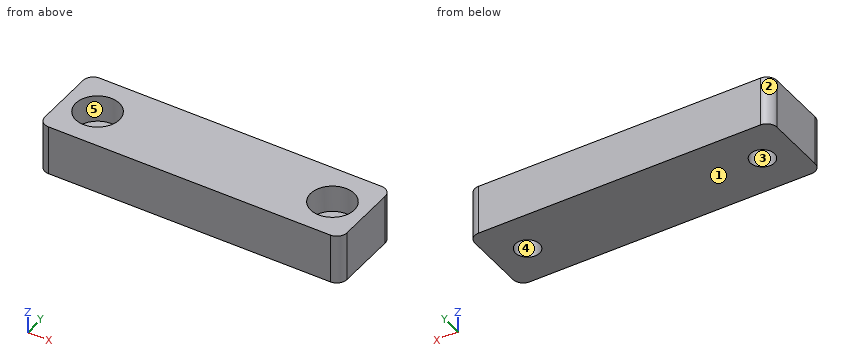
Solid Edge part; units mm, degrees
sketch "Sketch1" plane through (0, 0, 0) normal (0, 0, 1) x (1, 0, 0)
  line L0 (-22.5, 6) -> (-22.5, -6)
  line L1 (-22.5, -6) -> (22.5, -6)
  line L2 (22.5, -6) -> (22.5, 6)
  line L3 (22.5, 6) -> (-22.5, 6)
extrude "Protrusion1" add sketch "Sketch1" along normal blind 7.4
hole "Hole_1" at (17.5, 0, 7.4) direction (0, 0, -1) diameter 3.6 end through all counterbore diameter 6.5 counterbore depth 4
hole "Hole1" at (-17.5, 0, 7.4) direction (0, 0, -1) diameter 3.6 end through all counterbore diameter 6.5 counterbore depth 4
fillet "Round_1" radius 1.5 4 edges at (-22.5, -6, 3.7) (22.5, -6, 3.7) (22.5, 6, 3.7) (-22.5, 6, 3.7)
properties material "Acrylic, high impact grade"
Here's how the part is built. I have some questions about the finished solid (model axes, mm). Face numbers are marked on the shaded views. A direction names the side the tool comes from. Give positions to 0.01 mm unless a question says otherwise; leave off trailing zeros. Loops run counter-clockwise (first coordinate to the right, second up) from the corner with the lowest first, then second, coordinate; pieces in that order, holes last. Notation, with made-up numbers: M 61.5,-24 L 116.5,-24 A17 cw 116.5,-12 Z; hole C 25.5,73.5 d2. An arc over 180 degrees is marked long. Return JSON: item names as keys, results as strings.
Item 1: Imagine slicing it at C-C on x = 17.5. List the corners of the cut face in (y, z) for me, then the cut area to 3 significant figures.
A:
{"outline": "M -6,0 L -1.8,0 L -1.8,3.4 L -3.25,3.4 L -3.25,7.4 L -6,7.4 Z; M 1.8,0 L 6,0 L 6,7.4 L 3.25,7.4 L 3.25,3.4 L 1.8,3.4 Z", "area": "50.6 mm^2"}
Item 2: On a 3-axis mill with a long thin cutter (end or side, diameter ignored), from which of +Z, -Z, +X, -X, +Y, -Y can I reach the whole of each face in a straight line? I mean the marked faces 4 and 5. Say none if no direction works.
A:
{"face 4": "+Z, -Z", "face 5": "+Z"}
Item 3: I'm going to push flat-ended pins straight in: pin 1 Ø3 at (x, y) = (-17.5, 0) entering from +Z; pin 2 Ø4 at (x, y) = (-17.5, 0) entering from +Z. Where does each tip first touch, or does it pass through?
A:
{"pin 1": "passes through", "pin 2": "stops at z = 3.4"}
Item 4: Please list where these lines run through material, in increasing order: line 1 (X direction, y = 0, z = 4.5); line 2 (X direction, y = 0, z = 1.55); line 3 (Y direction, x = -17.5, z = 1.5).
A:
{"line 1": "x = -22.5 to -20.75, -14.25 to 14.25, 20.75 to 22.5", "line 2": "x = -22.5 to -19.3, -15.7 to 15.7, 19.3 to 22.5", "line 3": "y = -6 to -1.8, 1.8 to 6"}
Item 5: Thinking about a two-plate mould opening in Y: for the marked faces 1, 2 and 3, which applies, released by +Y, released by -Y, zero draft, split by the parting line, or undercut?
A:
{"face 1": "zero draft", "face 2": "released by +Y", "face 3": "undercut"}
Item 6: Imagine slicing it at D-D on z = 5. List the corners of the cut face in (x, y) for me.
A:
{"outline": "M -22.5,-4.5 A1.5 ccw -21,-6 L 21,-6 A1.5 ccw 22.5,-4.5 L 22.5,4.5 A1.5 ccw 21,6 L -21,6 A1.5 ccw -22.5,4.5 Z; hole C -17.5,0 d6.5; hole C 17.5,0 d6.5"}
Item 7: Imagine slicing it at B-B on z = 2.5. List the corners of the cut face in (x, y) for me, then the cut area to 3 significant figures.
A:
{"outline": "M -22.5,-4.5 A1.5 ccw -21,-6 L 21,-6 A1.5 ccw 22.5,-4.5 L 22.5,4.5 A1.5 ccw 21,6 L -21,6 A1.5 ccw -22.5,4.5 Z; hole C -17.5,0 d3.6; hole C 17.5,0 d3.6", "area": "518 mm^2"}
Item 8: Imagine slicing it at A-A on y = 0. List the corners of the cut face in (x, z) for me.
A:
{"outline": "M -22.5,0 L -19.3,0 L -19.3,3.4 L -20.75,3.4 L -20.75,7.4 L -22.5,7.4 Z; M -15.7,0 L 15.7,0 L 15.7,3.4 L 14.25,3.4 L 14.25,7.4 L -14.25,7.4 L -14.25,3.4 L -15.7,3.4 Z; M 19.3,0 L 22.5,0 L 22.5,7.4 L 20.75,7.4 L 20.75,3.4 L 19.3,3.4 Z"}
